Autodesk Inventor part; units mm, degrees
ref_plane "YZ Plane" through (0, 0, 0) normal (1, 0, 0) x (0, 1, 0)
ref_plane "XZ Plane" through (0, 0, 0) normal (0, 1, 0) x (-1, 0, 0)
ref_plane "XY Plane" through (0, 0, 0) normal (0, 0, 1) x (1, 0, 0)
sketch "Sketch2" plane through (0, 0, 0) normal (0, 0, 1) x (1, 0, 0)
  line L0 (109.6174, -113.2467) -> (109.6174, -116.2467)
  line L1 (106.6174, -113.2467) -> (106.6174, -116.2467)
  line L2 (101.6174, -113.2467) -> (109.6174, -113.2467)
  line L3 (101.6174, -116.2467) -> (109.6174, -116.2467)
  line L4 (101.6174, -113.2467) -> (101.6174, -116.2467)
  line L5 (106.6174, -113.2471) -> (106.6174, -108.2467)
  line L6 (109.6174, -113.2471) -> (109.6174, -108.2467)
  line L7 (106.6174, -108.2467) -> (106.6174, -98.2467)
  line L8 (109.6174, -108.2467) -> (109.6174, -98.2467)
  line L9 (109.6174, -98.2467) -> (109.6174, -88.2467)
  line L10 (106.6174, -98.2467) -> (106.6174, -88.2467)
  line L11 (106.6174, -88.2467) -> (106.6174, -78.2467)
  line L12 (109.6174, -88.2467) -> (109.6174, -78.2467)
  line L13 (109.6174, -78.2467) -> (109.6174, -68.2467)
  line L14 (106.6174, -78.2467) -> (106.6174, -68.2467)
  line L15 (106.6174, -78.2467) -> (109.6174, -78.2467)
  line L16 (106.6174, -88.2467) -> (109.6174, -88.2467)
  line L17 (106.6174, -98.2467) -> (109.6174, -98.2467)
  line L18 (106.6174, -108.2467) -> (109.6174, -108.2467)
  line L19 (91.6174, -113.2467) -> (91.6174, -116.2467)
  line L20 (81.6174, -113.2467) -> (81.6174, -116.2467)
  line L21 (71.6174, -113.2467) -> (71.6174, -116.2467)
  line L22 (61.6174, -113.2467) -> (61.6174, -116.2467)
  line L23 (51.6174, -113.2467) -> (51.6174, -116.2467)
  line L24 (106.6174, -68.2467) -> (109.6174, -68.2467)
  line L25 (109.6174, -108.2467) -> (106.6174, -108.2467)
  line L26 (109.6174, -98.2467) -> (106.6174, -98.2467)
  line L27 (109.6174, -88.2467) -> (106.6174, -88.2467)
  line L28 (109.6174, -78.2467) -> (106.6174, -78.2467)
  line L29 (101.6174, -113.2467) -> (101.6174, -116.2467)
  line L30 (91.6174, -113.2467) -> (91.6174, -116.2467)
  line L31 (81.6174, -113.2467) -> (81.6174, -116.2467)
  line L32 (71.6174, -113.2467) -> (71.6174, -116.2467)
  line L33 (61.6174, -113.2467) -> (61.6174, -116.2467)
  line L34 (51.6174, -113.2467) -> (51.6174, -116.2467)
  line L35 (106.6174, -113.2471) -> (106.6174, -113.2467)
  line L36 (106.6174, -113.2467) -> (106.6174, -113.2471)
  line L37 (109.6174, -108.2467) -> (109.6174, -113.2467)
  line L38 (106.6174, -98.2467) -> (106.6174, -108.2467)
  line L39 (106.6174, -108.2467) -> (106.6174, -98.2467)
  line L40 (106.6174, -88.2467) -> (106.6174, -78.2467)
  line L41 (109.6174, -68.2467) -> (109.6174, -78.2467)
  line L42 (109.6174, -88.2467) -> (109.6174, -98.2467)
  line L43 (106.6174, -78.2467) -> (106.6174, -88.2467)
  line L44 (101.6174, -113.2471) -> (106.6174, -113.2471)
  line L45 (101.6174, -116.2467) -> (91.6174, -116.2467)
  line L46 (61.6174, -113.2467) -> (71.6174, -113.2468)
  line L47 (81.6174, -113.2469) -> (91.6174, -113.247)
  line L48 (81.6174, -116.2467) -> (71.6174, -116.2467)
  line L49 (61.6174, -116.2467) -> (51.6174, -116.2467)
  line L50 (106.6174, -53.2467) -> (82.6898, -53.2467) construction
  line L51 (46.6174, -113.2467) -> (46.6174, -98.2467) construction
  line L52 (-8.3826, -113.2467) -> (-8.3826, -116.2467)
  line L53 (1.6174, -113.2467) -> (1.6174, -116.2467)
  line L54 (11.6174, -113.2467) -> (11.6174, -116.2467)
  line L55 (21.6174, -113.2467) -> (21.6174, -116.2467)
  line L56 (31.6174, -113.2467) -> (31.6174, -116.2467)
  line L57 (41.6174, -113.2467) -> (41.6174, -116.2467)
  line L58 (-8.3826, -113.2467) -> (-8.3826, -116.2467)
  line L59 (1.6174, -113.2467) -> (1.6174, -116.2467)
  line L60 (11.6174, -113.2467) -> (11.6174, -116.2467)
  line L61 (21.6174, -113.2467) -> (21.6174, -116.2467)
  line L62 (31.6174, -113.2467) -> (31.6174, -116.2467)
  line L63 (41.6174, -113.2467) -> (41.6174, -116.2467)
  line L64 (-8.3826, -116.2467) -> (1.6174, -116.2467)
  line L65 (11.6174, -116.2467) -> (21.6174, -116.2467)
  line L66 (31.6174, -116.2467) -> (41.6174, -116.2467)
  line L67 (-16.3826, -113.2471) -> (-16.3826, -108.2467)
  line L68 (-16.3826, -98.2467) -> (-16.3826, -88.2467)
  line L69 (-16.3826, -78.2467) -> (-16.3826, -68.2467)
  line L70 (-16.3826, -108.2467) -> (-16.3826, -113.2467)
  line L71 (-16.3826, -68.2467) -> (-16.3826, -78.2467)
  line L72 (-16.3826, -88.2467) -> (-16.3826, -98.2467)
  line L73 (109.6174, 6.7533) -> (109.6174, 6.7538)
  line L74 (106.6174, 6.7533) -> (106.6174, 6.7538)
  line L75 (101.6174, 6.7533) -> (109.6174, 6.7533)
  line L76 (101.6174, 6.7533) -> (101.6174, 9.7533)
  line L77 (106.6174, 6.7538) -> (106.6174, 6.7533)
  line L78 (109.6174, 6.7538) -> (109.6174, 1.7533)
  line L79 (106.6174, 1.7533) -> (106.6174, -8.2467)
  line L80 (109.6174, -8.2467) -> (109.6174, -18.2467)
  line L81 (106.6174, -18.2467) -> (106.6174, -28.2467)
  line L82 (109.6174, -28.2467) -> (109.6174, -38.2467)
  line L83 (106.6174, -28.2467) -> (109.6174, -28.2467)
  line L84 (106.6174, -18.2467) -> (109.6174, -18.2467)
  line L85 (106.6174, -8.2467) -> (109.6174, -8.2467)
  line L86 (106.6174, 1.7533) -> (109.6174, 1.7533)
  line L87 (91.6174, 6.7533) -> (91.6174, 9.7533)
  line L88 (81.6174, 6.7533) -> (81.6174, 9.7533)
  line L89 (71.6174, 6.7533) -> (71.6174, 9.7533)
  line L90 (61.6174, 6.7533) -> (61.6174, 9.7533)
  line L91 (51.6174, 6.7533) -> (51.6174, 9.7533)
  line L92 (106.6174, -38.2467) -> (109.6174, -38.2467)
  line L93 (109.6174, 1.7533) -> (106.6174, 1.7533)
  line L94 (109.6174, -8.2467) -> (106.6174, -8.2467)
  line L95 (109.6174, -18.2467) -> (106.6174, -18.2467)
  line L96 (109.6174, -28.2467) -> (106.6174, -28.2467)
  line L97 (101.6174, 6.7533) -> (101.6174, 9.7533)
  line L98 (91.6174, 6.7533) -> (91.6174, 9.7533)
  line L99 (81.6174, 6.7533) -> (81.6174, 9.7533)
  line L100 (71.6174, 6.7533) -> (71.6174, 9.7533)
  line L101 (61.6174, 6.7533) -> (61.6174, 9.7533)
  line L102 (51.6174, 6.7533) -> (51.6174, 9.7533)
  line L103 (106.6174, 6.7538) -> (106.6174, 6.7533)
  line L104 (106.6174, 6.7533) -> (106.6174, 6.7538)
  line L105 (109.6174, 1.7533) -> (109.6174, 6.7533)
  line L106 (106.6174, -8.2467) -> (106.6174, 1.7533)
  line L107 (106.6174, 1.7533) -> (106.6174, -8.2467)
  line L108 (106.6174, -18.2467) -> (106.6174, -28.2467)
  line L109 (109.6174, -38.2467) -> (109.6174, -28.2467)
  line L110 (109.6174, -18.2467) -> (109.6174, -8.2467)
  line L111 (106.6174, -28.2467) -> (106.6174, -18.2467)
  line L112 (101.6174, 6.7538) -> (106.6174, 6.7538)
  line L113 (101.6174, 9.7533) -> (91.6174, 9.7533)
  line L114 (61.6174, 6.7534) -> (71.6174, 6.7535)
  line L115 (81.6174, 6.7536) -> (91.6174, 6.7537)
  line L116 (81.6174, 9.7533) -> (71.6174, 9.7533)
  line L117 (61.6174, 9.7533) -> (51.6174, 9.7533)
  line L118 (46.6174, 6.7533) -> (46.6174, -8.2467) construction
  line L119 (31.6174, 6.7533) -> (31.6174, 9.7533)
  line L120 (41.6174, 6.7533) -> (41.6174, 9.7533)
  line L121 (31.6174, 6.7533) -> (31.6174, 9.7533)
  line L122 (41.6174, 6.7533) -> (41.6174, 9.7533)
  line L123 (31.6174, 9.7533) -> (41.6174, 9.7533)
  line L124 (-8.3826, 6.7533) -> (-8.3826, 9.7533)
  line L125 (1.6174, 6.7533) -> (1.6174, 9.7533)
  line L126 (11.6174, 6.7533) -> (11.6174, 9.7533)
  line L127 (21.6174, 6.7533) -> (21.6174, 9.7533)
  line L128 (-8.3826, 6.7533) -> (-8.3826, 9.7533)
  line L129 (1.6174, 6.7533) -> (1.6174, 9.7533)
  line L130 (-8.3826, 9.7533) -> (1.6174, 9.7533)
  line L131 (11.6174, 6.7533) -> (11.6174, 9.7533)
  line L132 (21.6174, 6.7533) -> (21.6174, 9.7533)
  line L133 (11.6174, 9.7533) -> (21.6174, 9.7533)
  line L134 (-16.3826, -8.2467) -> (-16.3826, -18.2467)
  line L135 (-16.3826, -18.2467) -> (-16.3826, -8.2467)
  line L136 (-16.3826, 1.7533) -> (-16.3826, 6.7533)
  line L137 (-16.3826, 6.7538) -> (-16.3826, 1.7533)
  line L138 (-16.3826, -28.2467) -> (-16.3826, -38.2467)
  line L139 (-16.3826, -38.2467) -> (-16.3826, -28.2467)
  line L140 (109.6174, -58.2467) -> (106.6174, -58.2467)
  line L141 (109.6174, -58.2467) -> (109.6174, -48.2467)
  line L142 (109.6174, -48.2467) -> (106.6174, -48.2467)
  line L143 (-16.3826, -68.2467) -> (-13.3826, -68.2467)
  line L144 (-16.3826, -58.2467) -> (-13.3826, -58.2467)
  line L145 (-16.3826, -58.2467) -> (-16.3826, -48.2467)
  line L146 (-16.3826, -48.2467) -> (-13.3826, -48.2467)
  line L147 (-16.3826, -38.2467) -> (-13.3826, -38.2467)
  line L148 (-16.3826, -108.2467) -> (-13.3826, -108.2467)
  line L149 (-16.3826, -98.2467) -> (-13.3826, -98.2467)
  line L150 (-16.3826, -88.2467) -> (-13.3826, -88.2467)
  line L151 (-16.3826, -78.2467) -> (-13.3826, -78.2467)
  line L152 (-16.3826, -28.2467) -> (-13.3826, -28.2467)
  line L153 (-16.3826, -18.2467) -> (-13.3826, -18.2467)
  line L154 (-16.3826, -8.2467) -> (-13.3826, -8.2467)
  line L155 (106.6174, -113.2467) -> (106.6174, -113.2471)
  line L156 (106.6174, -113.2471) -> (106.6174, -113.2467)
  line L157 (109.6174, -113.2467) -> (101.6174, -113.2467)
  line L158 (91.6174, -113.2467) -> (81.6174, -113.2467)
  line L159 (71.6174, -113.2467) -> (61.6174, -113.2467)
  line L160 (51.6174, -113.2467) -> (46.6174, -113.2467)
  line L161 (41.6174, -113.2467) -> (46.6174, -113.2467)
  line L162 (21.6174, -113.2467) -> (31.6174, -113.2467)
  line L163 (-16.3826, -113.2467) -> (-8.3826, -113.2467)
  line L164 (1.6174, -113.2467) -> (11.6174, -113.2467)
  line L165 (-13.3826, -98.2467) -> (-13.3826, -108.2467)
  line L166 (-13.3826, -108.2467) -> (-13.3826, -98.2467)
  line L167 (-13.3826, -88.2467) -> (-13.3826, -78.2467)
  line L168 (-13.3826, -78.2467) -> (-13.3826, -88.2467)
  line L169 (-13.3826, -58.2467) -> (-13.3826, -68.2467)
  line L170 (-13.3826, -68.2467) -> (-13.3826, -58.2467)
  line L171 (-13.3826, -48.2467) -> (-13.3826, -38.2467)
  line L172 (-13.3826, -38.2467) -> (-13.3826, -48.2467)
  line L173 (-13.3826, -18.2467) -> (-13.3826, -28.2467)
  line L174 (-13.3826, -28.2467) -> (-13.3826, -18.2467)
  line L175 (-16.3826, 1.7533) -> (-13.3826, 1.7533)
  line L176 (-13.3826, -8.2467) -> (-13.3826, 1.7533)
  line L177 (-13.3826, 1.7533) -> (-13.3826, -8.2467)
  line L178 (-16.3826, 6.7533) -> (-8.3826, 6.7533)
  line L179 (1.6174, 6.7533) -> (11.6174, 6.7533)
  line L180 (21.6174, 6.7533) -> (31.6174, 6.7533)
  line L181 (41.6174, 6.7533) -> (46.6174, 6.7533)
  line L182 (51.6174, 6.7533) -> (46.6174, 6.7533)
  line L183 (71.6174, 6.7533) -> (61.6174, 6.7533)
  line L184 (109.6174, 6.7533) -> (101.6174, 6.7533)
  line L185 (91.6174, 6.7533) -> (81.6174, 6.7533)
  line L186 (106.6174, 6.7533) -> (106.6174, 6.7538)
  line L187 (106.6174, 6.7538) -> (106.6174, 6.7533)
  line L188 (106.6174, 1.7533) -> (106.6174, -8.2467)
  line L189 (106.6174, -8.2467) -> (106.6174, 1.7533)
  line L190 (106.6174, -28.2467) -> (106.6174, -18.2467)
  line L191 (106.6174, -18.2467) -> (106.6174, -28.2467)
  line L192 (106.6174, -38.2467) -> (106.6174, -48.2467)
  line L193 (106.6174, -48.2467) -> (106.6174, -38.2467)
  line L194 (106.6174, -68.2467) -> (106.6174, -58.2467)
  line L195 (106.6174, -58.2467) -> (106.6174, -68.2467)
  line L196 (106.6174, -78.2467) -> (106.6174, -88.2467)
  line L197 (106.6174, -98.2467) -> (106.6174, -108.2467)
  line L198 (106.6174, -108.2467) -> (106.6174, -98.2467)
  line L199 (106.6174, -88.2467) -> (106.6174, -78.2467)
  point P0 (0, 0)
  point P1 (106.6174, -116.2467)
  point P2 (-13.3826, -113.2467)
extrude "Extrusion2" add sketch "Sketch2" along normal blind 3 contours L2 L5 L18 L6 | L2 L4 L45 L19 L47 L20 L48 L21 L46 L22 L49 L23 L160 L161 L57 L66 L56 L162 L55 L65 L54 L164 L53 L64 L52 L163 L67 L148 L165 L149 L68 L150 L167 L151 L69 L143 L169 L144 L145 L146 L171 L147 L138 L152 L173 L153 L134 L154 L176 L175 L136 L178 L124 L130 L125 L179 L126 L133 L127 L180 L119 L123 L120 L181 L182 L91 L117 L90 L114 L89 L116 L88 L115 L87 L113 L76 L75 L78 L86 L79 L85 L80 L84 L81 L83 L82 L92 L192 L142 L141 L140 L194 L14 L11 L10 L7 L5 | L17 L10 L16 L9 | L15 L14 L24 L13
sketch "Sketch3" plane through (0, 0, 3) normal (0, 0, 1) x (1, 0, 0)
  line L0 (51.6174, 4.7533) -> (51.6174, -111.2467)
  line L1 (51.6174, 4.7533) -> (48.6174, 4.7533)
  line L2 (41.6174, -113.2467) -> (51.6174, -113.2467)
  line L3 (51.6174, -113.2467) -> (51.6174, -53.2467)
  line L4 (51.6174, -53.2467) -> (48.6174, -53.2467)
  line L5 (48.6174, -53.2467) -> (48.6174, -8.2467)
  line L6 (48.6174, -8.2467) -> (51.6174, -8.2467)
  line L7 (48.6174, -53.2467) -> (48.6174, -98.2467)
  line L8 (48.6174, -98.2467) -> (51.6174, -98.2467)
  line L9 (51.6174, -98.2467) -> (51.6174, -8.2467)
  point P0 (0, 0)
  dimension "d20" = 60
  dimension "d21" = 45
  dimension "d22" = 45
extrude "Extrusion3" cut sketch "Sketch3" against normal blind 3
sketch "Sketch4" plane through (0, 0, 0) normal (0, 0, -1) x (-1, 0, 0)
  line L0 (-21.6174, -113.2467) -> (-31.6174, -113.2467)
  line L1 (13.3826, -58.2467) -> (13.3826, -68.2467)
  line L2 (-38.6174, -81.7467) -> (-38.6174, -84.7467)
  line L3 (-48.6174, -98.2467) -> (-48.6174, -8.2467)
  line L4 (-38.6174, -84.7467) -> (3.3826, -84.7467)
  circle A0 centre (-68.8966, -83.2467) radius 3
  line L5 (-38.6174, -81.7467) -> (3.3826, -81.7467)
  line L6 (3.3826, -81.7467) -> (3.3826, -84.7467)
  line L7 (13.3826, -78.2467) -> (13.3826, -88.2467)
  point P0 (0, 0)
  point P1 (-38.6174, -83.2467)
  dimension "d27" = 3
  dimension "d32" = 42
  dimension "d33" = 42
  dimension "d34" = 10
  dimension "d35" = 10
extrude "Extrusion4" cut sketch "Sketch4" against normal blind 10 contours L5 L6 L4 L2
properties part number "bottom"
Input: part model. Units: mm. Frame: model coordinates. A direction names the side the tool comes from. Coordinates: 2 decimals unless noted, no trailing zeros. Order: outer loops, then holes, each group sorted by start corner. A loop starts at its lowest first (then second) coordinate and runs counter-clockwise, first axis right, second up. Notation, with made-up numbers: M 21.25,0 L 30.25,0 A17 cw 30.25,12 Z; hole C 22,-2 d6. An arc over 180 degrees is marked long. Answer as CSV lines item,"result".
1. Section C-C (z = 1.75). State how many separate pieces and enclosed holes the cut face has, then the cut area to 3 significant figures.
Reported:
separate pieces,"1"
enclosed holes,"2"
area,"14,700 mm2"
2. Material intervals for line 1 (X direction, y = -82, z = 0.25); line 2 (X direction, y = -57, z = 2.6); line 3 (Y direction, x = 25, z = 1.2), sorted ascending. Write a range as from..to.
Reported:
line 1,"-13.38..-3.38, 38.62..48.62, 51.62..106.62"
line 2,"-16.38..48.62, 51.62..109.62"
line 3,"-113.25..-84.75, -81.75..6.75"
3. Section A-A (x = 36.5). Return the cut outline in (y, z).
Reported:
outline,"M -116.25,0 L -84.75,0 L -84.75,3 L -116.25,3 Z; M -81.75,0 L 9.75,0 L 9.75,3 L -81.75,3 Z"
4. Access query for faces 1 (the flat face through (106.617, -43, 1)), 2 (the flat face through (71.617, 8, 1)), 3 (the flat face through (-13.383, -23, 1)). Directions: +Z, -Z, +X, -X, +Y, -Y. A direction counts if a zero-diameter tool reaches every point of the face in a straight line with its end or side. Return the directions, or none.
Reported:
face 1,"+Z, -Z, +X"
face 2,"+Z, -Z, +Y"
face 3,"+Z, -Z, -X"
5. Section B-B (y = -20). Return the cut outline in (x, z), then the cut area to 3 significant figures.
Reported:
outline,"M -13.38,0 L 48.62,0 L 48.62,3 L -13.38,3 Z; M 51.62,0 L 106.62,0 L 106.62,3 L 51.62,3 Z"
area,"351 mm2"
6. Section D-D (x = 86). Return the cut outline in (y, z).
Reported:
outline,"M -113.25,0 L 6.75,0 L 6.75,3 L -113.25,3 Z"
7. First-contact query: P1, Ø1.5, axis at x = 50.5, z = 1.5, coming from the -Y side; P2, Ø1.5, axis at x = 26, z = 0.5, coming from the +Y side; P3, Ø1.5, axis at y = -114.5, z = 2, coming from the -X side. Flat tips, straight axial feed; report the tip coordinate or a pass-through.
Reported:
P1,"y = -113.25"
P2,"y = 6.75"
P3,"x = -8.38"
8. Pull-direction query (X, two-part tool) for faces 4 (the flat face through (50, -8.247, 2)), 5 (the flat face through (97, 9.753, 1)), 6 (the flat face through (109.617, -93, 1)); classes: released by +X, released by -X, zero draft, split by the parting line, or undercut.
Reported:
face 4,"undercut"
face 5,"zero draft"
face 6,"released by +X"
